```python
from build123d import *

# Parameters (mm, degrees)
BOSS_EXTRUDE1_DEPTH             = 300
SKETCH9_R                       = 2.5
BOSS_EXTRUDE2_DEPTH             = 3
BOSS_EXTRUDE3_DEPTH             = 9
BOSS_EXTRUDE3_DEPTH_BACK        = 9
SKETCH10_R                      = 21
SKETCH10_R_2                    = 17.5
CUT_EXTRUDE1_DEPTH              = 19
CUT_EXTRUDE1_DEPTH_BACK         = 19
F_3_0MM_DOWEL_HOLE1_D           = 3
F_3_0MM_DOWEL_HOLE1_DEPTH       = 7.5
F_3_0MM_DOWEL_HOLE1_CSINK_D     = 3.05
F_3_0MM_DOWEL_HOLE1_CSINK_ANGLE = 90
F_3_0MM_DOWEL_HOLE1_TIP         = 0.901290929
FILLET1_R                       = 5


with BuildPart() as part:
    # Sketch2 → Boss-Extrude1 (new body)
    with BuildSketch(Plane(origin=(0, 0, 0), x_dir=(0, 0, -1), z_dir=(1, 0, 0))):
        with BuildLine():
            Line((-8, 15), (8, 15))
            ThreePointArc((8, 15), (9.414213562, 14.414213562), (10, 13))
            Line((10, 13), (10, -13))
            ThreePointArc((10, -13), (9.414213562, -14.414213562), (8, -15))
            Line((8, -15), (-8, -15))
            ThreePointArc((-8, -15), (-9.414213562, -14.414213562), (-10, -13))
            Line((-10, -13), (-10, 13))
            ThreePointArc((-10, 13), (-9.414213562, 14.414213562), (-8, 15))
        make_face()
        with BuildLine():
            Line((-7, 14), (7, 14))
            ThreePointArc((7, 14), (8.414213562, 13.414213562), (9, 12))
            Line((9, 12), (9, -12))
            ThreePointArc((9, -12), (8.414213562, -13.414213562), (7, -14))
            Line((7, -14), (-7, -14))
            ThreePointArc((-7, -14), (-8.414213562, -13.414213562), (-9, -12))
            Line((-9, -12), (-9, 12))
            ThreePointArc((-9, 12), (-8.414213562, 13.414213562), (-7, 14))
        make_face(mode=Mode.SUBTRACT)
    extrude(amount=BOSS_EXTRUDE1_DEPTH)

    # Sketch9 → Boss-Extrude2 (add)
    # profile 1 of 2: a face of its own
    with BuildSketch(Plane(origin=(300, 0, 0), x_dir=(0, 0, -1), z_dir=(1, 0, 0))):
        with BuildLine():
            Line((0, -5), (0, -20))
            Line((0, -20), (30, -20))
            Line((30, -20), (30, 20))
            Line((30, 20), (0, 20))
            Line((0, 20), (0, 5))
            ThreePointArc((0, 5), (3.535533906, 3.535533906), (5, 0))
            ThreePointArc((5, 0), (3.535533906, -3.535533906), (0, -5))
        make_face()
        with Locations((23, -13)):
            Circle(SKETCH9_R, mode=Mode.SUBTRACT)
        with Locations((23, 13)):
            Circle(SKETCH9_R, mode=Mode.SUBTRACT)
    # profile 2 of 2: a face of its own
    with BuildSketch(Plane(origin=(300, 0, 0), x_dir=(0, 0, -1), z_dir=(1, 0, 0))):
        with BuildLine():
            Line((-30, 20), (-30, -20))
            Line((-30, -20), (0, -20))
            Line((0, -20), (0, -5))
            ThreePointArc((0, -5), (-5, 0), (0, 5))
            Line((0, 5), (0, 20))
            Line((0, 20), (-30, 20))
        make_face()
        with Locations((-23, -13)):
            Circle(SKETCH9_R, mode=Mode.SUBTRACT)
        with Locations((-23, 13)):
            Circle(SKETCH9_R, mode=Mode.SUBTRACT)
    extrude(amount=-BOSS_EXTRUDE2_DEPTH)

    # Sketch10 → Boss-Extrude3 (add, two sides: drawn at the far end of the back side and taken through both)
    # profile 1 of 3: a face of its own
    with BuildSketch(Plane.XY.offset(-BOSS_EXTRUDE3_DEPTH_BACK)):
        Circle(SKETCH10_R)
        Circle(SKETCH10_R_2, mode=Mode.SUBTRACT)
    # profile 2 of 3: a face of its own
    with BuildSketch(Plane.XY.offset(-BOSS_EXTRUDE3_DEPTH_BACK)):
        with BuildLine():
            ThreePointArc((9.013878189, 15), (0, 17.5), (-9.013878189, 15))
            Line((-9.013878189, 15), (9.013878189, 15))
        make_face()
    # profile 3 of 3: a face of its own
    with BuildSketch(Plane.XY.offset(-BOSS_EXTRUDE3_DEPTH_BACK)):
        with BuildLine():
            ThreePointArc((-9.013878189, -15), (0, -17.5), (9.013878189, -15))
            Line((9.013878189, -15), (-9.013878189, -15))
        make_face()
    extrude(amount=BOSS_EXTRUDE3_DEPTH + BOSS_EXTRUDE3_DEPTH_BACK)

    # Sketch10_3 → Cut-Extrude1 (cut, two sides: drawn at the far end of the back side and taken through both)
    with BuildSketch(Plane.XY.offset(-CUT_EXTRUDE1_DEPTH_BACK)):
        with BuildLine():
            Line((-9.013878189, -15), (9.013878189, -15))
            ThreePointArc((9.013878189, -15), (15.231429157, -8.617050879), (17.5, 0))
            ThreePointArc((17.5, 0), (15.231429157, 8.617050879), (9.013878189, 15))
            Line((9.013878189, 15), (-9.013878189, 15))
            ThreePointArc((-9.013878189, 15), (-17.5, 0), (-9.013878189, -15))
        make_face()
    extrude(amount=CUT_EXTRUDE1_DEPTH + CUT_EXTRUDE1_DEPTH_BACK, mode=Mode.SUBTRACT)

    # 3.0mm Dowel Hole1
    with Locations(Plane(origin=(0, -15, 0), x_dir=(1, 0, 0), z_dir=(0, 1, 0))):
        with Locations((0, 0)):
            CounterSinkHole(F_3_0MM_DOWEL_HOLE1_D / 2, F_3_0MM_DOWEL_HOLE1_CSINK_D / 2, depth=F_3_0MM_DOWEL_HOLE1_DEPTH, counter_sink_angle=F_3_0MM_DOWEL_HOLE1_CSINK_ANGLE)
            with Locations((0, 0, -(F_3_0MM_DOWEL_HOLE1_DEPTH + F_3_0MM_DOWEL_HOLE1_TIP / 2))):  # 118° drill point
                Cone(0, F_3_0MM_DOWEL_HOLE1_D / 2, F_3_0MM_DOWEL_HOLE1_TIP, mode=Mode.SUBTRACT)

    # Fillet1
    fillet1_edges = [part.edges().sort_by_distance(p)[0] for p in [
        (298.5, -20, 30),
        (298.5, 20, 30),
        (298.5, 20, -30),
        (298.5, -20, -30),
    ]]
    fillet(fillet1_edges, radius=FILLET1_R)


solid = part.part
```
Read the model definition and answer for the solid it produces. Units are mm, in the model's axes. A direction names the side the tool comes from. Give positions to 0.01 mm unless a question says otherwise; leave off trailing zeros. Write each loop counter-clockwise with the first axis right and the second up, starting at its lowest first coordinate (ties: lowest second). Pieces come first, ordered by that corner, then holes. Notation, with made-up numbers: (71, 20.25) -> (99, 20.25) arc R27 cw to (99, 40.25) -> close; hole circle Ø4 at (33.5, -6). An arc over 180 degrees is marked (long way). Answer as a JSON object with one key per item and string values.
1) Section A-A on x = 224 is taken. Write down the section's boundary in (y, z).
Findings below:
{"outline": "(-15, -8) arc R2 ccw to (-13, -10) -> (13, -10) arc R2 ccw to (15, -8) -> (15, 8) arc R2 ccw to (13, 10) -> (-13, 10) arc R2 ccw to (-15, 8) -> close; hole (-14, -7) arc R2 ccw to (-12, -9) -> (12, -9) arc R2 ccw to (14, -7) -> (14, 7) arc R2 ccw to (12, 9) -> (-12, 9) arc R2 ccw to (-14, 7) -> close"}
2) For a pull along Y with two mould halves and no side action, classify faces 1 (the flat face through (154, 15, 0)), 2 (the flat face through (154, -14, 0)), 3 (the flat face through (297, 0, 14)) as pulls with the +Y half, pulls with the -Y half, needs draft (parallel to the pull), parting line crosses it, or undercut.
Findings below:
{"face 1": "pulls with the +Y half", "face 2": "undercut", "face 3": "needs draft"}
3) Flat-ended cylindrical pins translate along their axes: pin 1 Ø10 at (x, z) = (248.5, -2) entering from +Y; pin 2 Ø11 at (x, z) = (147, -0.5) entering from -Y; pin 3 Ø7 at (x, y) = (208, -1.5) entering from +Z; pin 4 Ø8 at (y, z) = (13, -23) entering from +X. Find the tip coordinate at first contact, or state that the pin passes through.
Findings below:
{"pin 1": "stops at y = 15", "pin 2": "stops at y = -15", "pin 3": "stops at z = 10", "pin 4": "stops at x = 300"}
4) A tool of negligible diameter and unlimited length cuts with its end or side. For faces 4 (the flat face through (152, 0, -10)), 5 (the flat face through (154, -15, 0)), 6 (the flat face through (154, 14, 0)), 7 (the flat face through (0, -15, -2)), from which of +Z, -Z, +X, -X, +Y, -Y can it reach the whole face along a straight path? Write none if from no direction.
Findings below:
{"face 4": "-Z, -X, +Y, -Y", "face 5": "+Z, -Z, -Y", "face 6": "none", "face 7": "+Z, -Z"}
5) Section B-B on z = -14.5 is taken. Write down the section's boundary in (x, y), then the cut area to 3 significant figures.
Findings below:
{"outline": "(297, -20) -> (300, -20) -> (300, 20) -> (297, 20) -> close", "area": "120 mm^2"}
6) Straight lines are drawn through the part: probe 1 along Y at (x, z) = (298.25, 23); probe 2 along Z at (x, y) = (270.5, 6); probe 3 along Y at (x, z) = (79.5, -2.5). For each, find the intervals that lie inside material, in ascending order. Write a range as from..to.
Findings below:
{"probe 1": "y = -20..-15.5, -10.5..10.5, 15.5..20", "probe 2": "z = -10..-9, 9..10", "probe 3": "y = -15..-14, 14..15"}
